Could you check a few things on this model? Use its own coordinates, in mm. A direction names the side the tool comes from. Give positions to 0.01 mm unless a question says otherwise; leave off trailing zeros. Write each loop counter-clockwise with the first axis right and the second up, starting at its lowest first coordinate (ties: lowest second). Pieces come first, ordered by that corner, then holes. Notation, with made-up numbers: (89, 60.5) - (132, 60.5) arc R19 cw to (132, 67.5) - close; hole circle Ø10 at (-6, 58). An arc over 180 degrees is marked (long way). Answer in a Markdown table with one row per item.
Autodesk Fusion 360 part; units mm, degrees
sketch "Sketch1" plane through (0, 0, 0) normal (0, 0, 1) x (1, 0, 0) in component "Component"
  line L0 (0, 23.2) -> (86.2, 23.2) construction
  line L1 (86.2, 23.2) -> (86.2, 0) construction
  line L2 (86.2, 0) -> (0, 0) construction
  line L3 (0, 0) -> (0, 23.2) construction
  line L4 (86.2, 20.3) -> (82.8, 20.3)
  line L5 (82.8, 20.3) -> (82.8, 23.2)
  line L6 (82.8, 23.2) -> (63.2045, 23.2)
  line L7 (63.3, 23.2) -> (63.3, 20.8)
  line L8 (63.3, 20.8) -> (61.1, 20.8)
  line L9 (61.1, 20.8) -> (61.1, 23.2)
  line L10 (61.1, 23.2) -> (49.1, 23.2)
  line L11 (49.1, 23.2) -> (49.1, 18.6)
  line L12 (49.1, 18.6) -> (46.9, 18.6)
  line L13 (46.9, 18.6) -> (46.9, 23.2)
  line L14 (46.9, 23.2) -> (10, 23.2)
  line L15 (10, 23.2) -> (0, 18.2)
  line L16 (0, 18.2) -> (0, 5)
  line L17 (0, 5) -> (10, 0)
  line L18 (10, 0) -> (45, 0)
  line L19 (45, 0) -> (45, 2.6)
  line L20 (45, 2.6) -> (47.2, 2.6)
  line L21 (47.2, 2.6) -> (47.2, 0)
  line L22 (47.2, 0) -> (86.2, 0)
  line L23 (86.2, 0) -> (86.2, 20.3)
  circle A0 centre (25.2, 5) radius 2.5
  line L24 (78.4, 10.9318) -> (78.4, 4.2318)
  arc A1 (78.4, 4.2318) -> (81.9, 4.2318) centre (80.15, 4.2318) ccw
  line L25 (81.9, 4.2318) -> (81.9, 10.9318)
  arc A2 (81.9, 10.9318) -> (78.4, 10.9318) centre (80.15, 10.9318) ccw
  line L26 (55.1, 12) -> (54.6, 12)
  line L27 (54.6, 12) -> (54.6, 11)
  line L28 (54.6, 11) -> (55.1, 11)
  line L29 (55.1, 11) -> (55.1, 12)
  line L30 (74, 18.2) -> (74.5, 18.2)
  line L31 (74.5, 18.2) -> (74.5, 17.7)
  line L32 (74.5, 17.7) -> (74, 17.7)
  line L33 (74, 17.7) -> (74, 18.2)
  circle A3 centre (12.5, 11.6) radius 1
  line L34 (36.8702, 14.3809) -> (56.8702, 14.3809)
  line L35 (56.8702, 14.3809) -> (56.8702, 8.3809)
  line L36 (56.8702, 8.3809) -> (36.8702, 8.3809)
  line L37 (36.8702, 8.3809) -> (36.8702, 14.3809)
  line L38 (66.7799, 21.7291) -> (76.7799, 21.7291)
  line L39 (76.7799, 21.7291) -> (76.7799, 0.7291)
  line L40 (76.7799, 0.7291) -> (66.7799, 0.7291)
  line L41 (66.7799, 0.7291) -> (66.7799, 21.7291)
  dimension "d1" = 86.2
  dimension "d2" = 23.2
  dimension "d3" = 2.2
  dimension "d4" = 2.2
  dimension "d5" = 4.6
  dimension "d6" = 2.4
  dimension "d7" = 2.2
  dimension "d8" = 2.6
  dimension "d9" = 3.4
  dimension "d10" = 2.9
  dimension "d11" = 10
  dimension "d12" = 5
  dimension "d13" = 25.2
  dimension "d14" = 5
  dimension "d15" = 5
  dimension "d16" = 45
  dimension "d17" = 46.9
  dimension "d18" = 61.1
  dimension "d19" = 6.7
  dimension "d20" = 4.3
  dimension "d21" = 4.2318
  dimension "d22" = 1.75
  dimension "d23" = 0.5
  dimension "d24" = 55.1
  dimension "d25" = 1
  dimension "d26" = 12
  dimension "d27" = 0.5
  dimension "d28" = 0.5
  dimension "d29" = 74.5
  dimension "d30" = 5
  dimension "d33" = 80.15
  dimension "d34" = 2
  dimension "d35" = 12.5
  dimension "d36" = 11.6
  dimension "d48" = 20
  dimension "d49" = 6
  dimension "d50" = 10
  dimension "d51" = 21
extrude "Extrude1" add sketch "Sketch1" along normal blind 1.6 contours L4 L5 L6 L7 L8 L9 L10 L11 L12 L13 L14 L15 L16 L17 L18 L19 L20 L21 L22 L23 | L26 L27 L28 L29 | L30 L31 L32 L33 | A3 | L34 L35 L36 L37 | L38 L39 L40 L41 in component "Component"
extrude "Extrude2" cut sketch "Sketch1" along normal through all contours L26 L27 L28 L29 in component "Component"
extrude "Extrude3" cut sketch "Sketch1" along normal through all contours L30 L31 L32 L33 in component "Component"
pattern_linear "R-Pattern1" count 2 spacing 6.5 along (-1, 0, 0) count 4 spacing 4.5 along (0, -1, 0) of "Extrude3" in component "Component"
extrude "Extrude4" cut sketch "Sketch1" along normal through all contours A3 in component "Component"
pattern_linear "R-Pattern2" count 2 spacing 9.5 along (-1, 0, 0) of "Extrude2" in component "Component"
extrude "Extrude5" cut sketch "Sketch1" along normal blind 0.01 contours L34 L35 L36 L37 | L38 L39 L40 L41 in component "Component"
component "Component" placed x (1, 0, 0) y (0, 1, 0) z (0, 0, 1) at (0, 0, 0)
equation "d36 = d2 / 2"
1) Will this pin go through, and if not, where does the flat tip stop? P1, Ø1.6, axis at x = 12.5, y = 11.6, coming from the -Z side (3 decimals).
Check values:
| item | result |
|---|---|
| P1 | passes through |
2) Imagine slicing it at D-D (z = 1.3). State how many separate pieces and enclosed holes the cut face has, then the cut area to 3 significant figures.
Check values:
| item | result |
|---|---|
| separate pieces | 1 |
| enclosed holes | 13 |
| area | 1,860 mm2 |
3) If I drill on line 1 (Y direction, x = 12.5, z = 1.15); line 2 (X direction, y = 11.6, z = 0.5); line 3 (Y direction, x = 25.2, z = 0.95), over which ranges is the centre line in solid material (lowest first)?
Check values:
| item | result |
|---|---|
| line 1 | y = 0 to 10.6, 12.6 to 23.2 |
| line 2 | x = 0 to 11.5, 13.5 to 45.1, 45.6 to 54.6, 55.1 to 78.53, 81.77 to 86.2 |
| line 3 | y = 0 to 2.5, 7.5 to 23.2 |
4) Imagine slicing it at C-C (x = 80.15). List the corners of the cut face in (y, z) for me.
Check values:
| item | result |
|---|---|
| outline | (0, 0) - (2.48, 0) - (2.48, 1.6) - (0, 1.6) - close; (12.68, 0) - (23.2, 0) - (23.2, 1.6) - (12.68, 1.6) - close |
5) We'd pull the mould along Y, two halves only. Please class faces 1 (the face through (62, 20.8, 1)), 2 (the face through (33, 12, 0)), 3 (the face through (81.9, 8, 1)): +Y half, -Y half, draft (parallel to the pull), parting line (faces both ways), or undercut.
Check values:
| item | result |
|---|---|
| face 1 | +Y half |
| face 2 | draft |
| face 3 | undercut |
6) On a 3-axis mill with a long thin cutter (end or side, diameter ignored), from which of +Z, -Z, +X, -X, +Y, -Y can I reach the whole of each face in a straight line? I mean faces 4 (the face through (5.07, 20.735, 0.789)), 5 (the face through (82.8, 22, 1)), 6 (the face through (80.11, 12.68, 0.79)), 7 (the face through (63.3, 22, 1)). Say none if no direction works.
Check values:
| item | result |
|---|---|
| face 4 | +Z, -Z, -X, +Y |
| face 5 | +Z, -Z, +X, +Y |
| face 6 | +Z, -Z |
| face 7 | +Z, -Z, +Y |
7) Imagine slicing it at A-A (x = 12.5). List the corners of the cut face in (y, z) for me, then the cut area to 3 significant figures.
Check values:
| item | result |
|---|---|
| outline | (0, 0) - (10.6, 0) - (10.6, 1.6) - (0, 1.6) - close; (12.6, 0) - (23.2, 0) - (23.2, 1.6) - (12.6, 1.6) - close |
| area | 33.9 mm2 |
